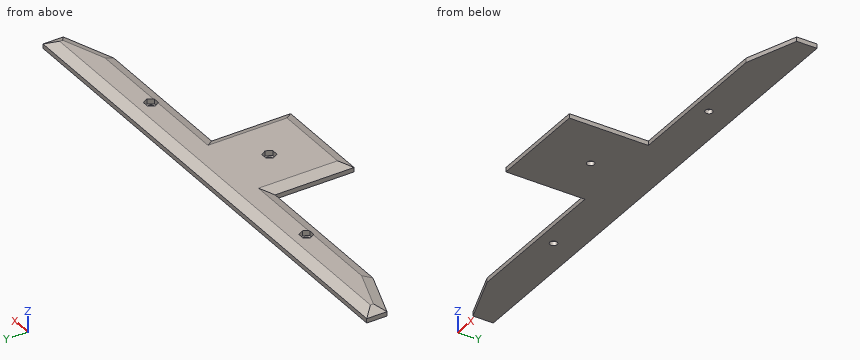
Solid Edge part; units mm, degrees
sketch "Sketch1" plane through (0, 0, 0) normal (0, 0, 1) x (1, 0, 0)
  line L0 (-125, 0) -> (125, 0)
  line L1 (125, -10) -> (125, 0)
  line L2 (100, -19) -> (125, -10)
  line L3 (-100, -19) -> (100, -19)
  line L4 (-125, -10) -> (-100, -19)
  line L5 (-125, 0) -> (-125, -10)
  dimension "D1" = 125
  dimension "D2" = 125
  dimension "D3" = 125
  dimension "D4" = 100
extrude "Protrusion1" add sketch "Sketch1" along normal blind 4.5
sketch "Sketch2" plane through (0, 0, 0) normal (0, 0, 1) x (1, 0, 0)
  line L0 (-24.5, -19) -> (24.5, -19)
  line L1 (24.5, -19) -> (24.5, -58)
  line L2 (24.5, -58) -> (-24.5, -58)
  line L3 (-24.5, -58) -> (-24.5, -19)
  dimension "D1" = 24.5
  dimension "D2" = 24.5
extrude "Extrusionsausprägung_2" add sketch "Sketch2" along normal blind 4.5
hole "Bohrung_1" at (-60, -11.8, 4.5) direction (0, 0, -1) diameter 3.6 end up to next
hole "Hole1" at (60, -11.8, 4.5) direction (0, 0, -1) diameter 3.6 end up to next
hole "Hole2" at (0, -31.8, 4.5) direction (0, 0, -1) diameter 3.6 end up to next
sketch "Sketch3" plane through (0, -29, 4.5) normal (0, 0, 1) x (1, 0, 0)
  line L0 (-61.5877, 19.95) -> (-63.1754, 17.2)
  line L1 (-63.1754, 17.2) -> (-61.5877, 14.45)
  line L2 (-61.5877, 14.45) -> (-58.4123, 14.45)
  line L3 (-58.4123, 14.45) -> (-56.8246, 17.2)
  line L4 (-56.8246, 17.2) -> (-58.4123, 19.95)
  line L5 (-58.4123, 19.95) -> (-61.5877, 19.95)
  line L6 (-1.5877, -0.05) -> (-3.1754, -2.8)
  line L7 (-3.1754, -2.8) -> (-1.5877, -5.55)
  line L8 (-1.5877, -5.55) -> (1.5877, -5.55)
  line L9 (1.5877, -5.55) -> (3.1754, -2.8)
  line L10 (3.1754, -2.8) -> (1.5877, -0.05)
  line L11 (1.5877, -0.05) -> (-1.5877, -0.05)
  line L12 (58.4123, 19.95) -> (56.8246, 17.2)
  line L13 (56.8246, 17.2) -> (58.4123, 14.45)
  line L14 (58.4123, 14.45) -> (61.5877, 14.45)
  line L15 (61.5877, 14.45) -> (63.1754, 17.2)
  line L16 (63.1754, 17.2) -> (61.5877, 19.95)
  line L17 (61.5877, 19.95) -> (58.4123, 19.95)
  dimension "D1" = 1.5877
  dimension "D2" = 61.5877
  dimension "D3" = 58.4123
extrude "Extrusionsausschnitt_1" cut sketch "Sketch3" against normal blind 2.5
chamfer "Fase_1" distance 5 angle 25 10 edges at (-62.25, -19, 4.5) (-24.5, -38.5, 4.5) (24.5, -38.5, 4.5) (0, -58, 4.5) (62.25, -19, 4.5) (112.5, -14.5, 4.5) (125, -5, 4.5) (0, 0, 4.5) (-125, -5, 4.5) (-112.5, -14.5, 4.5) measured on face at (85.8333, -9.0867, 4.5)
properties part number "54" material "Polyacticacid"
For this review, take the finished solid that the model builds, in its own axes (mm). Coordinates: 2 decimals unless noted, no trailing zeros. Write each loop counter-clockwise with the first axis right and the second up, starting at its lowest first coordinate (ties: lowest second). Pieces come first, ordered by that corner, then holes. Notation, with made-up numbers: (-4, -22) -> (9, -22) arc R22 ccw to (9, 9) -> close; hole circle Ø10 at (3.5, 35.5). An arc over 180 degrees is marked (long way). Write each question's results on one line, items separated by ' | '. Start each with the question number.
1) Insertion check: pin 1 (0.7 mm diameter, centred on x = 60, z = 3.5, fed in from +Y); pin 2 (4 mm diameter, centred on x = 60, y = -11.8, fed in from +Z); pin 3 (0.8 mm diameter, centred on x = -0.5, z = 3, fed in from +Y). Each pin has a flat end and moves straight along its axis. Give the tip position at first contact, or say it passes through.
2) Consider section B-B (x = -49). Write out the cut boundary in (y, z), plus the area to 3 significant figures.
3) Wall thickness on L1, parallel to X at y = -31.8, z = 0.55; L2, parallel to Y at x = 94.5, z = 0.85; L3, parallel to X at y = -23, z = 1.05: over which ranges is each line inside the solid? List them lowest first. Write a range as [from, to].
4) Consider section A-A (z = 2.85). Write out the cut boundary in (x, y), plus the area to 3 significant figures.
5) Consider section C-C (y = -40). Write out the cut boundary in (x, z), plus the area to 3 significant figures.
Geometry says:
1) pin 1: y = -2.1 | pin 2: z = 2 | pin 3: y = -0.93
2) outline: (-19, 0) -> (0, 0) -> (0, 2.17) -> (-5, 4.5) -> (-14, 4.5) -> (-19, 2.17) -> close | area: 73.8 mm^2
3) L1: [-24.5, -1.8], [1.8, 24.5] | L2: [-19, 0] | L3: [-24.5, 24.5]
4) outline: (-123.54, -8.97) -> (-99.74, -17.54) -> (-23.04, -17.54) -> (-23.04, -56.54) -> (23.04, -56.54) -> (23.04, -17.54) -> (99.74, -17.54) -> (123.54, -8.97) -> (123.54, -1.46) -> (-123.54, -1.46) -> close; hole (-63.18, -11.8) -> (-61.59, -14.55) -> (-58.41, -14.55) -> (-56.82, -11.8) -> (-58.41, -9.05) -> (-61.59, -9.05) -> close; hole (-3.18, -31.8) -> (-1.59, -34.55) -> (1.59, -34.55) -> (3.18, -31.8) -> (1.59, -29.05) -> (-1.59, -29.05) -> close; hole (56.82, -11.8) -> (58.41, -14.55) -> (61.59, -14.55) -> (63.18, -11.8) -> (61.59, -9.05) -> (58.41, -9.05) -> close | area: 5,490 mm^2
5) outline: (-24.5, 0) -> (24.5, 0) -> (24.5, 2.17) -> (19.5, 4.5) -> (-19.5, 4.5) -> (-24.5, 2.17) -> close | area: 209 mm^2
